Geometry: see drawing. Coordinates: mm, zero at the bounding-box minimum. Round coordinates to 2 decimals unless told otherwise and drop trailing zeros. Write each loop counter-clockwise with the first axis right and the second up, starting at its lowest first coordinate (ties: lowest second). Pieces come first, ordered by that corner, then holes. Notation, with made-up numbers: (48.25, 71.25) - (52.25, 71.25) arc R26 ccw to (52.25, 110.25) - close; hole circle Ø5 at (82, 40.5). An arc over 180 degrees is marked (long way). Use a Markdown table: item, result. Add a question column.
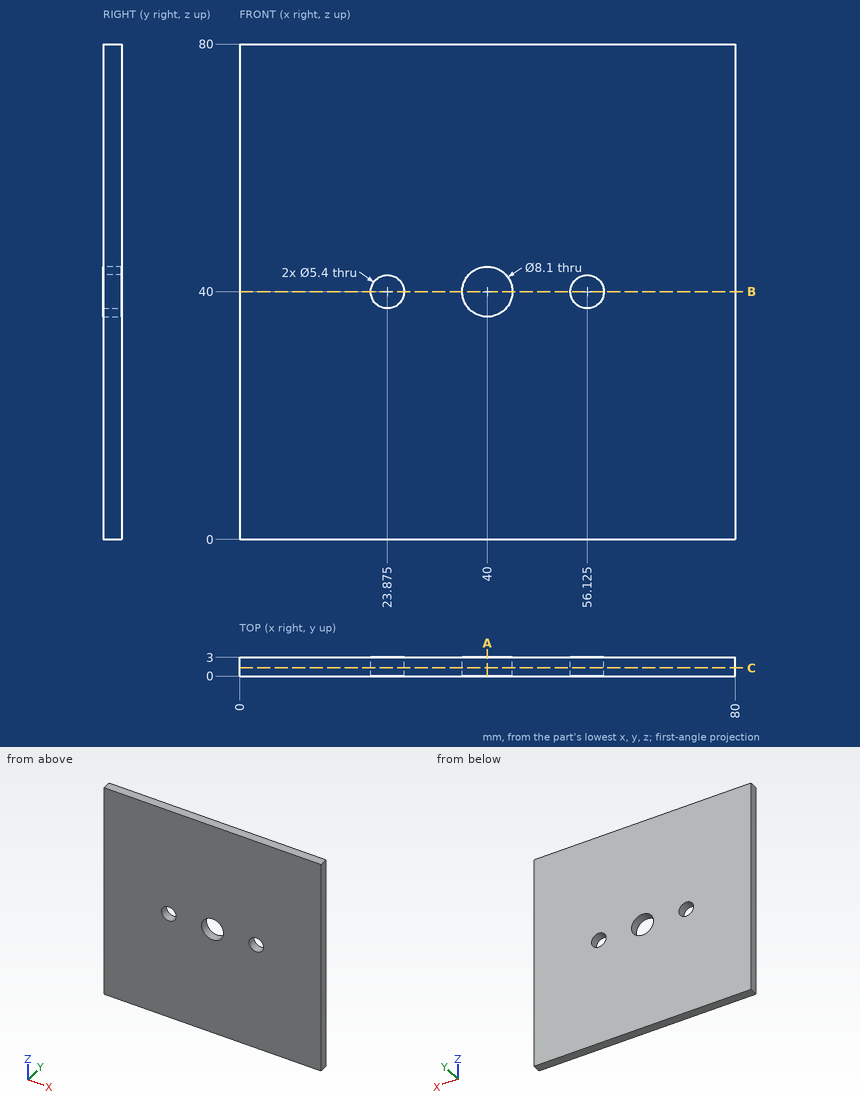
1) Section A-A, the plane x = 40. Return the cut outline in (y, z).
2) Section C-C, the plane y = 1.3. Return the cut outline in (x, z) (3 decimals), then the cut area to 3 significant figures.
3) Material intervals for L1, parallel to X at y = 1, z = 40 (3 decimals), sorted ascending. Write a range as from..to.
4) Section B-B, the plane z = 40. Return the cut outline in (x, y) (3 decimals), then the cut area to 3 significant figures.
Output values:
| question | item | result |
|---|---|---|
| 1 | outline | (0, 0) - (3, 0) - (3, 35.95) - (0, 35.95) - close; (0, 44.05) - (3, 44.05) - (3, 80) - (0, 80) - close |
| 2 | outline | (0, 0) - (80, 0) - (80, 80) - (0, 80) - close; hole circle Ø5.4 at (23.875, 40); hole circle Ø8.1 at (40, 40); hole circle Ø5.4 at (56.125, 40) |
| 2 | area | 6,300 mm^2 |
| 3 | L1 | x = 0..21.175, 26.575..35.95, 44.05..53.425, 58.825..80 |
| 4 | outline | (0, 0) - (21.175, 0) - (21.175, 3) - (0, 3) - close; (26.575, 0) - (35.95, 0) - (35.95, 3) - (26.575, 3) - close; (44.05, 0) - (53.425, 0) - (53.425, 3) - (44.05, 3) - close; (58.825, 0) - (80, 0) - (80, 3) - (58.825, 3) - close |
| 4 | area | 183 mm^2 |
